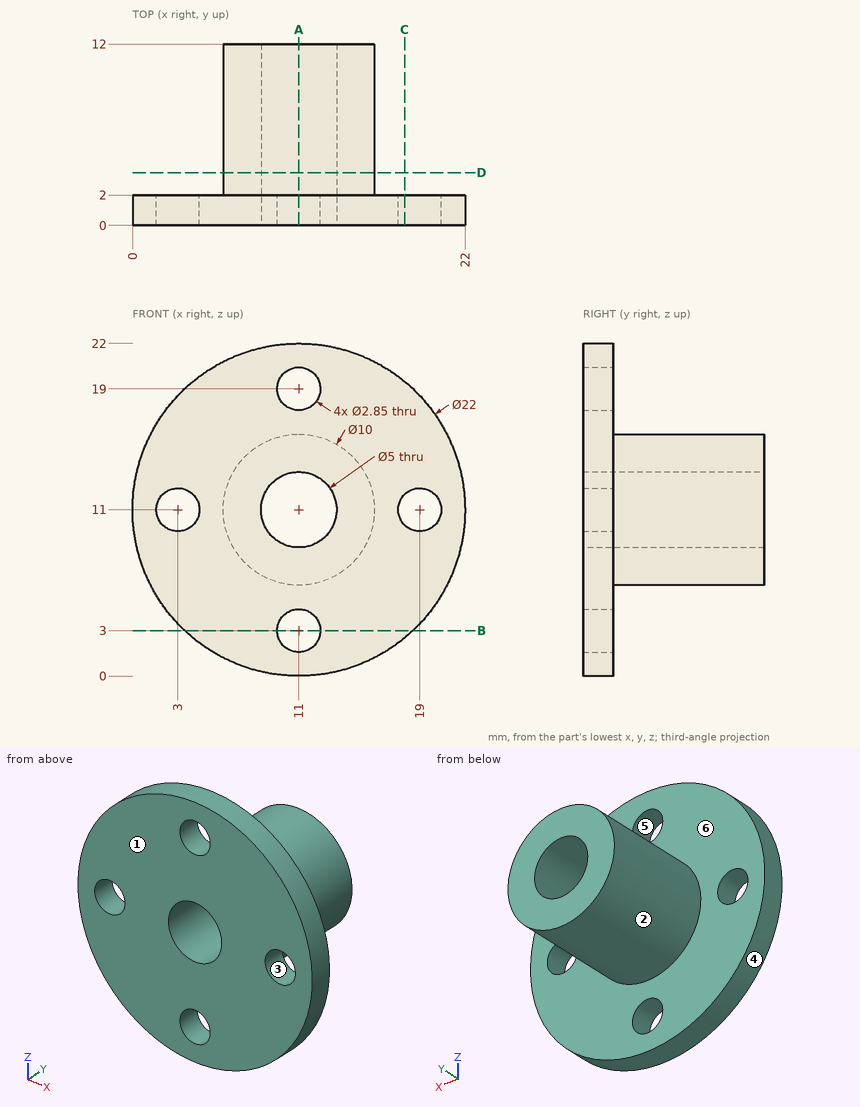
Geometry: see drawing. Coordinates: mm, zero at the bounding-box minimum. A direction names the side the tool comes from. Coordinates: 2 decimals unless noted, no trailing zeros. Write each loop counter-clockwise with the first axis right and the second up, starting at its lowest first coordinate (ties: lowest second). Pieces come first, ordered by that corner, then holes. Notation, with made-up numbers: M 79,21 L 114,21 A17 ccw 114,26 Z; hole C 85,36 d9. An arc over 180 degrees is marked long. Use CSV: the item, a comma, the result in double quotes. Start each with the question number.
1. First-contact query: P1, Ø6, axis at y = 7.5, z = 18, coming from the -X side; P2, Ø2.5, axis at x = 19, z = 11, coming from the +Y side; P3, Ø5, axis at y = 5.5, z = 12.5, coming from the +X side; P4, Ø4, axis at x = 5, y = 2, coming from the -Z side. Flat tips, straight axial feed; report the tip coordinate or a pass-through.
2. Reachability of the marked faces 1 and 2 from +Z, -Z, +X, -X, +Y, -Y: full face, straight path, thin tool, end or side. Return the list, or none.
3. Cut plane D-D on y = 3.5. Return the cut outline in (x, z).
4. Mould query, pull axis Z, two halves, no side actions, for the marked faces 3, 4, 5 and 6. Classes: pulls with the +Z half, pulls with the -Z half, needs draft (parallel to the pull), parting line crosses it, or undercut.
5. Cut plane C-C on x = 18. Return the cut outline in (y, z).
6. Cut plane B-B on z = 3. Return the cut outline in (x, y) (3 decimals).
7. Cut plane A-A on x = 11. Return the cut outline in (y, z) (3 decimals).
8. Ray query, probe 1 along X at (y, z) = (2.5, 11); probe 2 along Y at (x, z) = (20.25, 8); probe 3 along X at (y, z) = (1.05, 19) (3 decimals). Return the intervals inside material, ascending.
Entries:
1,P1,"x = 8"
1,P2,"through"
1,P3,"x = 16"
1,P4,"z = 0.75"
2,face 1,"+Z, -Z, +X, -X, -Y"
2,face 2,"+Y"
3,outline,"C 11,11 d10; hole C 11,11 d5"
4,face 3,"undercut"
4,face 4,"parting line crosses it"
4,face 5,"undercut"
4,face 6,"needs draft"
5,outline,"M 0,2.51 L 2,2.51 L 2,9.98 L 0,9.98 Z; M 0,12.02 L 2,12.02 L 2,19.49 L 0,19.49 Z"
6,outline,"M 3.45,0 L 9.575,0 L 9.575,2 L 3.45,2 Z; M 12.425,0 L 18.55,0 L 18.55,2 L 12.425,2 Z"
7,outline,"M 0,0 L 2,0 L 2,1.575 L 0,1.575 Z; M 0,4.425 L 2,4.425 L 2,6 L 12,6 L 12,8.5 L 0,8.5 Z; M 0,13.5 L 12,13.5 L 12,16 L 2,16 L 2,17.575 L 0,17.575 Z; M 0,20.425 L 2,20.425 L 2,22 L 0,22 Z"
8,probe 1,"6 to 8.5, 13.5 to 16"
8,probe 2,"0 to 2"
8,probe 3,"3.45 to 9.575, 12.425 to 18.55"
